Autodesk Inventor part; units mm, degrees
ref_plane "YZ Plane" through (0, 0, 0) normal (1, 0, 0) x (0, 1, 0)
ref_plane "XZ Plane" through (0, 0, 0) normal (0, 1, 0) x (-1, 0, 0)
ref_plane "XY Plane" through (0, 0, 0) normal (0, 0, 1) x (1, 0, 0)
sketch "Sketch1" plane through (0, 0, 0) normal (0, 0, 1) x (1, 0, 0)
  circle A0 centre (0, 0) radius 5
  line L0 (-42.5, 35) -> (42.5, 35)
  line L1 (42.5, 35) -> (42.5, -35)
  line L2 (42.5, -35) -> (-42.5, -35)
  line L3 (-42.5, -35) -> (-42.5, 35)
  line L4 (42.5, 35) -> (-42.5, -35) construction
  line L5 (0, 15) -> (0, -15)
  circle A1 centre (-32.5, 25) radius 5
  circle A2 centre (32.5, 25) radius 5
  circle A3 centre (-32.5, -25) radius 5
  circle A4 centre (32.5, -25) radius 5
  dimension "d0" = 10
  dimension "d1" = 70
  dimension "d2" = 85
  dimension "d3" = 15
  dimension "d4" = 30
  dimension "d5" = 10
  dimension "d6" = 10
  dimension "d7" = 10
  dimension "d8" = 10
  dimension "d11" = 65
extrude "Extrusion1" add sketch "Sketch1" along normal blind 15
properties part number "dudukan u bolt" material "Steel, Mild"
Verification items for the finished model (mm, model axes). Round coordinates to 2 decimals unless told otherwise and drop trailing zeros. Write each loop counter-clockwise with the first axis right and the second up, starting at its lowest first coordinate (ties: lowest second). Pieces come first, ordered by that corner, then holes. Notation, with made-up numbers: (-39, -8) -> (15, -8) arc R28 ccw to (15, 27) -> close; hole circle Ø5 at (-15.5, -0.75). An arc over 180 degrees is marked (long way). Write each question's results on one line, items separated by ' | '. Start each with the question number.
1. Cross-section at A-A (x = 0). Enter the section's corners in (y, z).
2. Cross-section at D-D (y = 25). Enter the section's corners in (x, z).
3. Cross-section at B-B (z = 12.5). Enter the section's corners in (x, y).
4. Draft check along X on faces 1 (the flat face through (1, -35, 7)), 2 (the cylindrical face through (-36.5, -22, 7.4)), 3 (the flat face through (42.5, 0, 7)). Enter one of: +X half, -X half, draft (parallel to the pull), parting line (faces both ways), or undercut.
5. Material ranges on probe 1 along Y at (x, z) = (32.5, 5.25); probe 2 along X at (y, z) = (-21.5, 5.25); probe 3 along Y at (x, z) = (31, 2.75), recorded low to high. Write a range as from..to.
6. Depth check by flat-ended pin: P1, Ø6, axis at x = 0, y = 0, coming from the +Z side. Enter the tip coordinate at first touch or a pass-through.
7. Cross-section at C-C (x = -32.5). Enter the section's corners in (y, z), then the cut area to 3 significant figures.
Solutions:
1) outline: (-35, 0) -> (-5, 0) -> (-5, 15) -> (-35, 15) -> close; (5, 0) -> (35, 0) -> (35, 15) -> (5, 15) -> close
2) outline: (-42.5, 0) -> (-37.5, 0) -> (-37.5, 15) -> (-42.5, 15) -> close; (-27.5, 0) -> (27.5, 0) -> (27.5, 15) -> (-27.5, 15) -> close; (37.5, 0) -> (42.5, 0) -> (42.5, 15) -> (37.5, 15) -> close
3) outline: (-42.5, -35) -> (42.5, -35) -> (42.5, 35) -> (-42.5, 35) -> close; hole circle Ø10 at (-32.5, -25); hole circle Ø10 at (-32.5, 25); hole circle Ø10 at (0, 0); hole circle Ø10 at (32.5, -25); hole circle Ø10 at (32.5, 25)
4) face 1: draft | face 2: undercut | face 3: +X half
5) probe 1: y = -35..-30, -20..20, 30..35 | probe 2: x = -42.5..-36.07, -28.93..28.93, 36.07..42.5 | probe 3: y = -35..-29.77, -20.23..20.23, 29.77..35
6) P1: passes through
7) outline: (-35, 0) -> (-30, 0) -> (-30, 15) -> (-35, 15) -> close; (-20, 0) -> (20, 0) -> (20, 15) -> (-20, 15) -> close; (30, 0) -> (35, 0) -> (35, 15) -> (30, 15) -> close | area: 750 mm2
